The model under review builds one solid part; all positions refer to its coordinate system, in mm. Coordinates: 2 decimals unless noted, no trailing zeros. Order: outer loops, then holes, each group sorted by start corner. A loop starts at its lowest first (then second) coordinate and runs counter-clockwise, first axis right, second up. Notation, with made-up numbers: (-2, 53.25) -> (33, 53.25) arc R4 ccw to (33, 58.25) -> close; hole circle Ø8 at (19, 38). An arc over 180 degrees is marked (long way). Put each result on its own line as item: value.
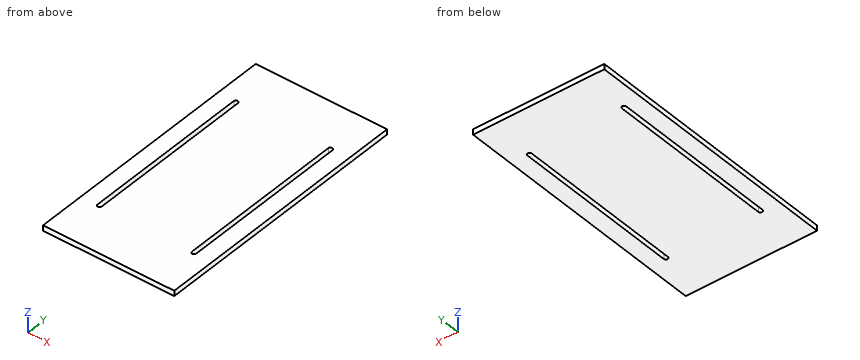
from build123d import *

# Parameters (mm, degrees)
SKETCH1_W            = 50
SKETCH1_H            = 100
BOSS_EXTRUDE1_DEPTH  = 2
CUT_EXTRUDE1_DEPTH   = 56.937465084
LPATTERN1_COUNT      = 2
LPATTERN1_PITCH      = 36
MIRROR1_COPY_1_DEPTH = 56.937465084


with BuildPart() as part:
    # Sketch1 → Boss-Extrude1 (new body)
    with BuildSketch(Plane.XY):
        Rectangle(SKETCH1_W, SKETCH1_H)
    extrude(amount=BOSS_EXTRUDE1_DEPTH)

    # Sketch2 → Cut-Extrude1 (cut, through all)
    with BuildSketch(Plane(origin=(0, 0, 0), x_dir=(-1, 0, 0), z_dir=(0, 0, -1))):
        with BuildLine():
            Line((-18.8, 0), (-17.2, 0))
            Line((-17.2, 0), (-17.2, 32.021950636))
            ThreePointArc((-17.2, 32.021950636), (-18, 32.821950636), (-18.8, 32.021950636))
            Line((-18.8, 32.021950636), (-18.8, 0))
        make_face()
    cut_extrude1 = extrude(amount=-CUT_EXTRUDE1_DEPTH, mode=Mode.SUBTRACT)

    # LPattern1: Cut-Extrude1 ×2
    with Locations(*[(-i * LPATTERN1_PITCH, 0, 0) for i in range(1, LPATTERN1_COUNT)]):
        add(cut_extrude1, mode=Mode.SUBTRACT)

    # Mirror1: Cut-Extrude1 across plane
    add(cut_extrude1.mirror(Plane.ZX), mode=Mode.SUBTRACT)

    # Mirror1 copy 1 sketch → Mirror1 copy 1 (cut, through all)
    with BuildSketch(Plane(origin=(-36, 0, 0), x_dir=(-1, 0, 0), z_dir=(0, 0, -1))):
        with BuildLine():
            Line((-18.8, 0), (-17.2, 0))
            Line((-17.2, 0), (-17.2, -32.021950636))
            ThreePointArc((-17.2, -32.021950636), (-18, -32.821950636), (-18.8, -32.021950636))
            Line((-18.8, -32.021950636), (-18.8, 0))
        make_face()
    extrude(amount=-MIRROR1_COPY_1_DEPTH, mode=Mode.SUBTRACT)


solid = part.part
Item 1: Consider section B-B on z = 1.05. Write out the cut boundary in (x, y).
Answers below:
outline: (-25, -50) -> (25, -50) -> (25, 50) -> (-25, 50) -> close; hole (-18.8, -32.02) arc R0.8 ccw to (-17.2, -32.02) -> (-17.2, 32.02) arc R0.8 ccw to (-18.8, 32.02) -> close; hole (17.2, -32.02) arc R0.8 ccw to (18.8, -32.02) -> (18.8, 32.02) arc R0.8 ccw to (17.2, 32.02) -> close
Item 2: For line 1 (X direction, y = 11, z = 0.8); line 2 (Y direction, x = -18.5, z = 0.9), list the stretches that pass through material, from the lowest coordinate up. Write a range as from..to.
Answers below:
line 1: -25..-18.8, -17.2..17.2, 18.8..25
line 2: -50..-32.65, 32.65..50
Item 3: Consider section A-A on y = -8.5. Write out the cut boundary in (x, z), and give its area (3 significant figures).
Answers below:
outline: (-25, 0) -> (-18.8, 0) -> (-18.8, 2) -> (-25, 2) -> close; (-17.2, 0) -> (17.2, 0) -> (17.2, 2) -> (-17.2, 2) -> close; (18.8, 0) -> (25, 0) -> (25, 2) -> (18.8, 2) -> close
area: 93.6 mm^2
